Source: CAD feature listing. Evaluate the final solid. Frame: model axes, mm. A direction names the side the tool comes from. Give positions to 0.01 mm unless a question says otherwise; leave off trailing zeros. Write each loop counter-clockwise with the first axis right and the second up, starting at its lowest first coordinate (ties: lowest second). Pieces come first, ordered by that corner, then holes.
```python
from build123d import *

# Parameters (mm, degrees)
F0_R     = 1.5
F1_DEPTH = 2.7
F2_DEPTH = 3.2
F3_DEPTH = 2.7
F4_DEPTH = 3.2
F5_DEPTH = 1.7
F6_DEPTH = 3.2


with BuildPart() as f1:
    # F0 (on Top) → F1 (new body)
    with BuildSketch(Plane.XY):
        with BuildLine():
            Line((-4.325, 2.1857004834), (-4.325, -1.4937755356))
            ThreePointArc((-4.325, -1.4937755356), (-2.6690400274, -1.7468749135), (-1.1504704305, -2.4541295388))
            ThreePointArc((-1.1504704305, -2.4541295388), (-1.0926241638, -2.4923454544), (-1.0352298419, -2.5312368234))
            ThreePointArc((-1.0352298419, -2.5312368234), (-0.263537277, -2.8804262246), (0.575, -3))
            Line((0.575, -3), (3.975, -2.6046511628))
            Line((3.975, -2.6046511628), (3.975, 4.6964450739))
            Line((3.975, 4.6964450739), (1.5472968315, 4.6964450739))
            add(Edge.make_bspline(
                [(1.5472968315, 4.6964450739), (1.3144459312, 4.3733731641), (0.6967900923, 3.6911224637), (0.1028413655, 3.3605125255), (-0.240789904, 3.1692369025)],
                knots=[0.6540594598, 0.6540594598, 0.6540594598, 0.6540594598, 0.7998547995, 1, 1, 1, 1], degree=3))
            Line((-0.240789904, 3.1692369025), (-4.325, 2.1857004834))
        make_face()
        with Locations((0.575, 0)):
            Circle(F0_R, mode=Mode.SUBTRACT)
    extrude(amount=F1_DEPTH)

    # F0 (on Top) → F2 (join)
    with BuildSketch(Plane.XY):
        with BuildLine():
            Line((-11.325, 0.5), (-11.325, -3))
            Line((-11.325, -3), (-8.325, -3))
            ThreePointArc((-8.325, -3), (-6.4658219239, -1.872914493), (-4.325, -1.4937755356))
            Line((-4.325, -1.4937755356), (-4.325, 2.1857004834))
            Line((-4.325, 2.1857004834), (-11.325, 0.5))
        make_face()
    extrude(amount=F2_DEPTH)

    # F0 (on Top) → F3 (join)
    with BuildSketch(Plane.XY):
        with BuildLine():
            add(Edge.make_bspline(
                [(2.1125420716, 5.6967418641), (2.0793732606, 5.6176202325), (1.9227685724, 5.2694923337), (1.7196807638, 4.9356213286), (1.5472968315, 4.6964450739)],
                knots=[0.5147370924, 0.5147370924, 0.5147370924, 0.5147370924, 0.546124408, 0.6540594598, 0.6540594598, 0.6540594598, 0.6540594598], degree=3))
            Line((1.5472968315, 4.6964450739), (3.975, 4.6964450739))
            Line((3.975, 4.6964450739), (3.975, 5.6967418641))
            Line((3.975, 5.6967418641), (2.1125420716, 5.6967418641))
        make_face()
        with BuildLine():
            add(Edge.make_bspline(
                [(2.975, 10), (2.8586448523, 9.1762784971), (2.6455796583, 7.6679104943), (2.3594416082, 6.2857016012), (2.1125420716, 5.6967418641)],
                knots=[0, 0, 0, 0, 0.2810985188, 0.5147370924, 0.5147370924, 0.5147370924, 0.5147370924], degree=3))
            Line((2.1125420716, 5.6967418641), (3.975, 5.6967418641))
            Line((3.975, 5.6967418641), (3.975, 15))
            Line((3.975, 15), (0.9666787216, 10.1831827385))
            Line((0.9666787216, 10.1831827385), (2.975, 10))
        make_face()
    extrude(amount=F3_DEPTH)

    # F0 (on Top) → F4 (join)
    with BuildSketch(Plane.XY):
        with BuildLine():
            Line((3.975, 15), (3.975, 5.6967418641))
            Line((3.975, 5.6967418641), (6.3370948682, 5.6967418641))
            ThreePointArc((6.3370948682, 5.6967418641), (5.9175559365, 6.8145730008), (5.775, 8))
            Line((5.775, 8), (5.775, 15))
            Line((5.775, 15), (3.975, 15))
        make_face()
        with BuildLine():
            Line((3.975, 5.6967418641), (3.975, 4.6964450739))
            Line((3.975, 4.6964450739), (7.0217980536, 4.6964450739))
            ThreePointArc((7.0217980536, 4.6964450739), (6.6490204546, 5.1757668667), (6.3370948682, 5.6967418641))
            Line((6.3370948682, 5.6967418641), (3.975, 5.6967418641))
        make_face()
        with BuildLine():
            Line((7.0217980536, 4.6964450739), (3.975, 4.6964450739))
            Line((3.975, 4.6964450739), (3.975, -2.6046511628))
            Line((3.975, -2.6046511628), (11.325, -1.75))
            Line((11.325, -1.75), (11.325, 2.9936889187))
            Line((11.325, 2.9936889187), (11.325, 3))
            Line((11.325, 3), (11.3100688905, 3))
            Line((11.3100688905, 3), (10.775, 3))
            ThreePointArc((10.775, 3), (8.7156038058, 3.4438078053), (7.0217980536, 4.6964450739))
        make_face()
    extrude(amount=F4_DEPTH)

    # F0 (on Top) → F5 (join)
    with BuildSketch(Plane.XY):
        with BuildLine():
            Line((3.975, 15), (3.975, 5.6967418641))
            Line((3.975, 5.6967418641), (6.3370948682, 5.6967418641))
            ThreePointArc((6.3370948682, 5.6967418641), (5.9175559365, 6.8145730008), (5.775, 8))
            Line((5.775, 8), (5.775, 15))
            Line((5.775, 15), (3.975, 15))
        make_face()
        with BuildLine():
            add(Edge.make_bspline(
                [(2.975, 10), (2.8586448523, 9.1762784971), (2.6455796583, 7.6679104943), (2.3594416082, 6.2857016012), (2.1125420716, 5.6967418641)],
                knots=[0, 0, 0, 0, 0.2810985188, 0.5147370924, 0.5147370924, 0.5147370924, 0.5147370924], degree=3))
            Line((2.1125420716, 5.6967418641), (3.975, 5.6967418641))
            Line((3.975, 5.6967418641), (3.975, 15))
            Line((3.975, 15), (0.9666787216, 10.1831827385))
            Line((0.9666787216, 10.1831827385), (2.975, 10))
        make_face()
    extrude(amount=-F5_DEPTH)

    # F0 (on Top) → F6 (join)
    with BuildSketch(Plane.XY):
        with BuildLine():
            Line((7.0217980536, 4.6964450739), (3.975, 4.6964450739))
            Line((3.975, 4.6964450739), (3.975, -2.6046511628))
            Line((3.975, -2.6046511628), (11.325, -1.75))
            Line((11.325, -1.75), (11.325, 2.9936889187))
            Line((11.325, 2.9936889187), (11.325, 3))
            Line((11.325, 3), (11.3100688905, 3))
            Line((11.3100688905, 3), (10.775, 3))
            ThreePointArc((10.775, 3), (8.7156038058, 3.4438078053), (7.0217980536, 4.6964450739))
        make_face()
    extrude(amount=F6_DEPTH)


solid = f1.part
```
1. Section query B-B (x = 3.25). Return loops of the section in (y, z), plus the area to 3 significant figures.
2. Pull-direction query (X, two-part tool) for faces 4 (the cylindrical face through (-0.27, -2.88, 1.33)), 5 (the flat face through (-11.325, -1, 2)), 6 (the flat face through (7, 2, 3.2)); classes: pulls with the +X half, pulls with the -X half, needs draft (parallel to the pull), parting line crosses it, or undercut.
3. Pin query (flat end, axial travel): P1, Ø7, axis at x = -5.5, y = 1, coming from the -Z side; P2, Ø0.8, axis at x = 5, z = -1, coming from the -Y side; P3, Ø8, axis at x = -0.5, y = 4.5, coming from the +Z side. Return the tip coordinate at first contact, or that it passes through.
4. Section query D-D (x = -5.75). Return loops of the section in (y, z).
5. Access query for faces 1 (the flat face through (2.4, 0.4, 0)), 2 (the flat face through (1, 2, 2.7)), 3 (the flat face through (5.775, 11, 1)). Directions: +Z, -Z, +X, -X, +Y, -Y. A direction counts if a zero-diameter tool reaches every point of the face in a straight line with its end or side. Return the directions, or none.
6. Line query: probe 1 along Z at (x, y) = (-4.75, -0.5); probe 2 along X at (y, z) = (12.5, 2.9) (3 decimals); probe 3 along Z at (x, y) = (3.25, 10.75). Output: solid intervals per line, ascending.
7. Section query A-A (y = 0). Return loops of the section in (x, z) (3 decimals), plus the area to 3 significant figures.
8. Section query C-C (y = 13). Return loops of the section in (x, z) (3 decimals).
The answers:
1. outline: (-2.69, 0) - (5.7, 0) - (5.7, -1.7) - (13.84, -1.7) - (13.84, 2.7) - (-2.69, 2.7) - close
1. area: 58.5 mm2
2. face 4: undercut
2. face 5: pulls with the -X half
2. face 6: needs draft
3. P1: stops at z = 0
3. P2: stops at y = 5.7
3. P3: stops at z = 2.7
4. outline: (-1.65, 0) - (1.84, 0) - (1.84, 3.2) - (-1.65, 3.2) - close
5. face 1: -Z, +X, -X, -Y
5. face 2: +Z, +Y, -Y
5. face 3: +Z, -Z, +X, +Y
6. probe 1: z = 0 to 3.2
6. probe 2: x = 3.975 to 5.775
6. probe 3: z = -1.7 to 2.7
7. outline: (-11.325, 0) - (-0.925, 0) - (-0.925, 2.7) - (-4.325, 2.7) - (-4.325, 3.2) - (-11.325, 3.2) - close; (2.075, 0) - (11.325, 0) - (11.325, 3.2) - (3.975, 3.2) - (3.975, 2.7) - (2.075, 2.7) - close
7. area: 60.2 mm2
8. outline: (2.726, -1.7) - (5.775, -1.7) - (5.775, 3.2) - (3.975, 3.2) - (3.975, 2.7) - (2.726, 2.7) - close
